Read the model definition and answer for the solid it produces. Units are mm, in the model's axes. A direction names the side the tool comes from. Round coordinates to 2 decimals unless told otherwise and drop trailing zeros. Loops run counter-clockwise (first coordinate to the right, second up) from the corner with the lowest first, then second, coordinate; pieces in that order, holes last. Notation, with made-up numbers: M -28,40.25 L -22,40.25 A8 cw -22,47.25 Z; hole C 74.25,89.5 d6. An arc over 180 degrees is marked long. Write each question's results on one line, items separated by ' | '.
Autodesk Inventor part; units mm, degrees
ref_plane "YZ Plane" through (0, 0, 0) normal (1, 0, 0) x (0, 1, 0)
ref_plane "XZ Plane" through (0, 0, 0) normal (0, 1, 0) x (-1, 0, 0)
ref_plane "XY Plane" through (0, 0, 0) normal (0, 0, 1) x (1, 0, 0)
sketch "Sketch1" plane through (0, 0, 0) normal (0, 0, 1) x (1, 0, 0)
  line L0 (0, 0) -> (44.45, 0)
  line L1 (44.45, 0) -> (44.45, 25.4)
  line L2 (44.45, 25.4) -> (0, 25.4)
  line L3 (0, 25.4) -> (0, 0)
  circle A0 centre (12.7, 12.7) radius 2.413
  line L4 (0, 12.7) -> (44.45, 12.7) construction
  circle A1 centre (38.1, 12.7) radius 2.413
  dimension "d0" = 44.45
  dimension "d1" = 25.4
  dimension "d2" = 4.826
  dimension "d6" = 25.4
  dimension "d32" = 6.35
extrude "Plate1" add sketch "Sketch1" along normal blind 3.175
sketch "Sketch2" plane through (0, 26.67, 4.445) normal (0, 1, 0) x (-1, 0, 0)
  line L0 (-44.45, 0) -> (0, 0)
  line L1 (0, 0) -> (0, 33.655)
  line L2 (0, 33.655) -> (-44.45, 33.655)
  line L3 (-44.45, 33.655) -> (-44.45, 0)
edge flange "Flange1" height 38.1 angle 90 thickness 3.175 bend radius 1.27 thickness toward (0, 1, 0) relief tear relief width 3.175 relief depth 1.5875 edges at (22.225, 25.4, 3.175) wall of the first edge with corners at (44.45, 26.67, 4.445) (0, 26.67, 4.445) (0, 26.67, 38.1) (44.45, 26.67, 38.1)
bend "Bend1"
corner "Corner1"
fillet "Fillet1" radius 1.5875 4 edges at (44.45, 0, 1.5875) (0, 0, 1.5875) (44.45, 28.2575, 38.1) (0, 28.2575, 38.1)
sketch "Sketch3" plane through (0, 26.67, 4.445) normal (0, -1, 0) x (1, 0, 0)
  line L0 (3.175, 33.655) -> (22.225, 33.655) construction
  line L1 (22.225, 33.655) -> (22.225, -0.635) construction
  line L2 (22.225, -0.635) -> (3.175, -0.635) construction
  line L3 (3.175, -0.635) -> (3.175, 33.655) construction
  circle A0 centre (19.05, 27.9019) radius 2.413
  line L4 (12.7, 33.655) -> (12.7, -0.635) construction
  line L5 (3.175, 16.51) -> (22.225, 16.51) construction
  circle A1 centre (6.35, 27.9019) radius 2.413
  circle A2 centre (19.05, 5.1181) radius 2.413
  circle A3 centre (6.35, 5.1181) radius 2.413
  line L6 (44.45, 32.0675) -> (44.45, 0)
  line L7 (42.8625, 33.655) -> (1.5875, 33.655)
  point P0 (0, -4.445)
  dimension "d23" = 34.29
  dimension "d24" = 19.05
  dimension "d27" = 4.826
  dimension "d28" = 3.175
  dimension "d29" = 5.7531
  dimension "d33" = 22.225
extrude "Extrusion1" cut sketch "Sketch3" against normal blind 25.4
equation "\"d12\" = BendReliefWidth"
equation "\"d13\" = BendReliefDepth"
equation "\"d14\" = MinimumRemnant"
equation "\"d15\" = BendRadius"
equation "\"d19\" = CornerReliefSize"
equation "\"d20\" = GapSize"
equation "\"d21\" = JacobiRadiusSize"
equation "\"BendRadius\" = Thickness"
equation "\"BendReliefWidth\" = Thickness"
equation "\"BendReliefDepth\" = 0.5 * Thickness"
equation "\"CornerReliefSize\" = 4 * Thickness"
equation "\"MinimumRemnant\" = 2 * Thickness"
equation "\"TransitionRadius\" = BendRadius"
equation "\"JacobiRadiusSize\" = BendRadius"
equation "\"GapSize\" = Thickness"
equation "\"d11\" = BendRadius"
properties part number "Pneumatic Piston Back Flange (Rt Custom)"
1. Find section D-D, the plane z = 30.5. Give the vertices of the cut face in (x, y) (3 decimals).
Completed:
outline: M 0,26.67 L 4.797,26.67 L 4.797,29.845 L 0,29.845 Z; M 7.903,26.67 L 17.497,26.67 L 17.497,29.845 L 7.903,29.845 Z; M 20.603,26.67 L 44.45,26.67 L 44.45,29.845 L 20.603,29.845 Z
2. Given P1, Ø6, axis at x = 25, y = 10.5, coming from the +Z side (3 decimals); P2, Ø8, axis at x = 38.5, z = 20, coming from the -Y side, each flat-ended and moving along its own axis, determine where each tip first touches the part or whether it passes through.
Completed:
P1: stops at z = 3.175 | P2: stops at y = 26.67
3. Find section A-A, the plane x = 19.05. Give the vertices of the cut face in (y, z) (3 decimals), then the cut area to 3 significant figures.
Completed:
outline: M 0,0 L 25.4,0 A4.445 ccw 29.845,4.445 L 29.845,7.15 L 26.67,7.15 L 26.67,4.445 A1.27 cw 25.4,3.175 L 0,3.175 Z; M 26.67,11.976 L 29.845,11.976 L 29.845,29.934 L 26.67,29.934 Z; M 26.67,34.76 L 29.845,34.76 L 29.845,38.1 L 26.67,38.1 Z | area: 171 mm2
4. Find the intervals of material crossed by L1, parallel to Z at x = 19.05, y = 28.5; L2, parallel to Y at x = 30, z = 17 (3 decimals); L3, parallel to Z at x = 17, y = 25.25 (3 decimals), in increasing order.
Completed:
L1: z = 1.26 to 7.15, 11.98 to 29.93, 34.76 to 38.1 | L2: y = 26.67 to 29.845 | L3: z = 0 to 3.175
5. Which of the six approach directions +Z, -Z, +X, -X, +Y, -Y give full straight-line access (tool end or side, diameter ignored) to faces 5 (the face through (22, 13, 3.175)), 6 (the face through (0.45, 0.48, 1.61))?
Completed:
face 5: +Z, +X, -X, -Y | face 6: +Z, -Z, -X, -Y
6. Find section B-B, the plane y = 12.7. Give the vertices of the cut face in (x, z) (3 decimals), then the cut area to 3 significant figures.
Completed:
outline: M 0,0 L 10.287,0 L 10.287,3.175 L 0,3.175 Z; M 15.113,0 L 35.687,0 L 35.687,3.175 L 15.113,3.175 Z; M 40.513,0 L 44.45,0 L 44.45,3.175 L 40.513,3.175 Z | area: 110 mm2
7. Find section C-C, the plane x = 38.1. Give the vertices of the cut face in (y, z) (3 decimals).
Completed:
outline: M 0,0 L 10.287,0 L 10.287,3.175 L 0,3.175 Z; M 15.113,0 L 25.4,0 A4.445 ccw 29.845,4.445 L 29.845,38.1 L 26.67,38.1 L 26.67,4.445 A1.27 cw 25.4,3.175 L 15.113,3.175 Z
8. Determine the mould class of faces 1 (the face through (43.97, 0.45, 1.61)), 2 (the face through (8.65, 28.24, 10.29)), 3 (the face through (0.45, 28.28, 37.62)), 4 (the face through (21.91, 26.31, 3.56)) for opening direction X: released by +X, released by -X, zero draft, split by the parting line, or undercut.
Completed:
face 1: released by +X | face 2: undercut | face 3: released by -X | face 4: zero draft
